```python
from build123d import *

# Parameters (mm, degrees)
CROQUIS1_W              = 260
CROQUIS1_H              = 150
SALIENTE_EXTRUIR1_DEPTH = 4
CROQUIS2_R              = 2.6
CROQUIS2_W              = 124
CROQUIS2_H              = 70
CORTAR_EXTRUIR1_DEPTH   = 4
CROQUIS3_R              = 1.6
CORTAR_EXTRUIR2_DEPTH   = 10


with BuildPart() as part:
    # Croquis1 → Saliente-Extruir1 (new body)
    with BuildSketch(Plane(origin=(0, 0, 0), x_dir=(1, 0, 0), z_dir=(0, 1, 0))):
        Rectangle(CROQUIS1_W, CROQUIS1_H)
    extrude(amount=SALIENTE_EXTRUIR1_DEPTH)

    # Croquis2 → Cortar-Extruir1 (cut)
    with BuildSketch(Plane(origin=(0, 4, 0), x_dir=(1, 0, 0), z_dir=(0, 1, 0))):
        with Locations(Location((-115, 60, 0), (0, 0, 270))):
            Circle(CROQUIS2_R)
        with Locations(Location((115, 60, 0), (0, 0, 270))):
            Circle(CROQUIS2_R)
        with Locations(Location((115, -50, 0), (0, 0, 270))):
            Circle(CROQUIS2_R)
        with Locations(Location((-115, -50, 0), (0, 0, 270))):
            Circle(CROQUIS2_R)
        with Locations((0, 40)):
            Rectangle(CROQUIS2_W, CROQUIS2_H)
    extrude(amount=-CORTAR_EXTRUIR1_DEPTH, mode=Mode.SUBTRACT)

    # Croquis3 → Cortar-Extruir2 (cut)
    with BuildSketch(Plane(origin=(0, 4, 0), x_dir=(1, 0, 0), z_dir=(0, 1, 0))):
        with Locations(Location((95, -55, 0), (0, 0, 270))):
            Circle(CROQUIS3_R)
        with Locations(Location((-95, -55, 0), (0, 0, 270))):
            Circle(CROQUIS3_R)
    extrude(amount=-CORTAR_EXTRUIR2_DEPTH, mode=Mode.SUBTRACT)


solid = part.part
```
Verification items for the finished model (mm, model axes). Coordinates: 2 decimals unless noted, no trailing zeros. Order: outer loops, then holes, each group sorted by start corner. A loop starts at its lowest first (then second) coordinate and runs counter-clockwise, first axis right, second up. Notation, with made-up numbers: (7.5, 44.5) -> (28.5, 44.5) arc R15 cw to (28.5, 62.5) -> close; hole circle Ø7 at (47, -37.75). An arc over 180 degrees is marked (long way). Put each result on its own line as item: value. Start each with the question number.
1) Go/stop test with a flat-tipped pin: pin 1 (12 mm diameter, centred on x = -10, z = 22, fed in from -Y). Record where the tip stops, or that it passes through.
2) Cross-section at D-D (z = -29.5). Enter the section's corners in (x, y).
3) Material ranges on L1, parallel to X at y = 2.35, z = -60; L2, parallel to X at y = 1.35, z = -43; L3, parallel to X at y = 2.75, z = 55, recorded low to high.
4) Cross-section at A-A (z = -60). Enter the section's corners in (x, y), plus the area to 3 significant figures.
5) Release check for a two-part mould opening along Z. For faces 1 (the cylindrical face through (116.757, 2.028, -61.916)), 2 (the flat face through (-2, 4, 16)) record: pulls with the +Z half, pulls with the -Z half, needs draft (parallel to the pull), parting line crosses it, or undercut.
6) Cross-section at C-C (z = 50). Enter the section's corners in (x, y), plus the area to 3 significant figures.
7) Cross-section at B-B (y = 2.45). Enter the section's corners in (x, z).
Geometry check:
1. pin 1: stops at y = 0
2. outline: (-130, 0) -> (-62, 0) -> (-62, 4) -> (-130, 4) -> close; (62, 0) -> (130, 0) -> (130, 4) -> (62, 4) -> close
3. L1: x = -130 to -117.6, -112.4 to -62, 62 to 112.4, 117.6 to 130
3. L2: x = -130 to -62, 62 to 130
3. L3: x = -130 to -96.6, -93.4 to 93.4, 96.6 to 130
4. outline: (-130, 0) -> (-117.6, 0) -> (-117.6, 4) -> (-130, 4) -> close; (-112.4, 0) -> (-62, 0) -> (-62, 4) -> (-112.4, 4) -> close; (62, 0) -> (112.4, 0) -> (112.4, 4) -> (62, 4) -> close; (117.6, 0) -> (130, 0) -> (130, 4) -> (117.6, 4) -> close
4. area: 502 mm^2
5. face 1: undercut
5. face 2: needs draft
6. outline: (-130, 0) -> (-117.6, 0) -> (-117.6, 4) -> (-130, 4) -> close; (-112.4, 0) -> (112.4, 0) -> (112.4, 4) -> (-112.4, 4) -> close; (117.6, 0) -> (130, 0) -> (130, 4) -> (117.6, 4) -> close
6. area: 998 mm^2
7. outline: (-130, -75) -> (-62, -75) -> (-62, -5) -> (62, -5) -> (62, -75) -> (130, -75) -> (130, 75) -> (-130, 75) -> close; hole circle Ø5.2 at (-115, -60); hole circle Ø5.2 at (-115, 50); hole circle Ø3.2 at (-95, 55); hole circle Ø3.2 at (95, 55); hole circle Ø5.2 at (115, -60); hole circle Ø5.2 at (115, 50)
